Could you check a few things on this drawing? It's one solid part, dimensions in mm from its lowest x, y, z. Round coordinates to 2 decimals unless told otherwise and drop trailing zeros. Loops run counter-clockwise (first coordinate to the right, second up) from the corner with the lowest first, then second, coordinate; pieces in that order, holes last. Notation, with made-up numbers: (41.5, 11) -> (72.5, 11) arc R30 ccw to (72.5, 49) -> close; hole circle Ø11 at (-15, 21.25). An arc over 180 degrees is marked (long way). Write each question's results on one line, items separated by ' | '.
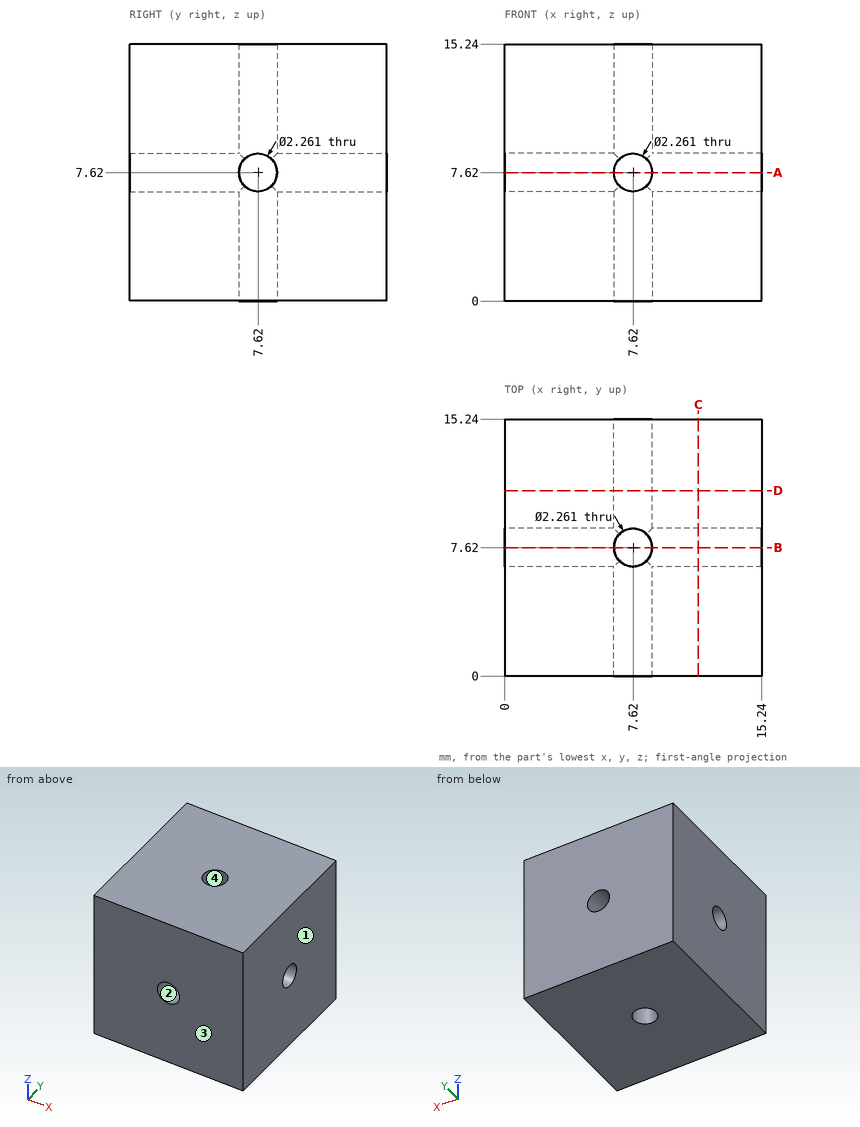
1) I want a section at A-A, the plane z = 7.62. Write out the boundary of the cut face in (x, y).
Model answer:
outline: (0, 0) -> (6.49, 0) -> (6.49, 6.49) -> (0, 6.49) -> close; (0, 8.75) -> (6.49, 8.75) -> (6.49, 15.24) -> (0, 15.24) -> close; (8.75, 0) -> (15.24, 0) -> (15.24, 6.49) -> (8.75, 6.49) -> close; (8.75, 8.75) -> (15.24, 8.75) -> (15.24, 15.24) -> (8.75, 15.24) -> close
2) I need wall thicknesses on line 1 (Z direction, x = 10.75, y = 7.62); line 2 (Z direction, x = 7.75, y = 11); line 3 (X direction, y = 1.5, z = 7) (1 decimal). Which ranges of each line are inside material? Lowest first, please.
Model answer:
line 1: z = 0 to 6.49, 8.75 to 15.24 | line 2: z = 0 to 6.5, 8.74 to 15.24 | line 3: x = 0 to 6.7, 8.6 to 15.2
3) If we mould it in two halves opening along X, with no side actions, what happens to the marked faces 1, 2, 3 and 4? For each: released by +X, released by -X, zero draft, split by the parting line, or undercut.
Model answer:
face 1: released by +X | face 2: undercut | face 3: zero draft | face 4: undercut
4) I want a section at C-C, the plane x = 11.5. Write out the boundary of the cut face in (y, z).
Model answer:
outline: (0, 0) -> (15.24, 0) -> (15.24, 15.24) -> (0, 15.24) -> close; hole circle Ø2.26 at (7.62, 7.62)
5) I'm going to push a flat-ended pin straight in: pin 1 (3.5 mm diameter, centred on x = 7.62, y = 7.62, fed in from -Z). Where does the tip first touch, or does it pass through?
Model answer:
pin 1: stops at z = 0
